For this review, take the finished solid that the model builds, in its own axes (mm). Face numbers are marked on the shaded views. A direction names the side the tool comes from. Round coordinates to 2 decimals unless told otherwise and drop trailing zeros. Order: outer loops, then holes, each group sorted by start corner. A loop starts at its lowest first (then second) coordinate and runs counter-clockwise, first axis right, second up. Notation, with made-up numbers: (47.5, -34) - (90.5, -34) arc R17 ccw to (90.5, -2) - close; hole circle Ø4 at (42, 52). An arc over 180 degrees is marked (long way). One line per question, with ' | ' between items.
```python
from build123d import *

# Parameters (mm, degrees)
SKETCH_1_R                   = 15
EXTRUDE_1_DEPTH              = 5
SKETCH_1_5_R                 = 12
SKETCH_1_5_R_2               = 9.125
EXTRUDE_2_DEPTH              = 20
HOLE_WIZARD_M3_1_D           = 3.4
HOLE_WIZARD_M3_1_CSINK_D     = 6.6
HOLE_WIZARD_M3_1_CSINK_ANGLE = 90
SKETCH1_R                    = 3.25
CUT_EXTRUDE1_DEPTH           = 16
CUT_EXTRUDE1_DEPTH_BACK      = 16
M3_CLEARANCE_HOLE1_D         = 3.4
M3_CLEARANCE_HOLE1_DEPTH     = 35
M3_CLEARANCE_HOLE1_TIP       = 1.021463052


with BuildPart() as part:
    # 草图1 → 凸台-拉伸1 (new body)
    with BuildSketch(Plane(origin=(0, 0, 0), x_dir=(0, 0, -1), z_dir=(1, 0, 0))):
        Circle(SKETCH_1_R)
    extrude(amount=EXTRUDE_1_DEPTH)

    # 草图1<5> → 凸台-拉伸2 (add)
    with BuildSketch(Plane(origin=(0, 0, 0), x_dir=(0, 0, -1), z_dir=(1, 0, 0))):
        Circle(SKETCH_1_5_R)
        Circle(SKETCH_1_5_R_2, mode=Mode.SUBTRACT)
    extrude(amount=EXTRUDE_2_DEPTH)

    # M3 十字槽沉头木螺钉的锥形沉头孔1 (through all)
    with Locations(Plane(origin=(5, 0, 0), x_dir=(0, 0, 1), z_dir=(1, 0, 0))):
        with Locations((0, -5), (-5, 0), (0, 5), (5, 0)):
            CounterSinkHole(HOLE_WIZARD_M3_1_D / 2, HOLE_WIZARD_M3_1_CSINK_D / 2, counter_sink_angle=HOLE_WIZARD_M3_1_CSINK_ANGLE)

    # Sketch1 → Cut-Extrude1 (cut, two sides)
    with BuildSketch(Plane.XY) as cut_extrude1_sk:
        with Locations((12.5, 0)):
            Circle(SKETCH1_R)
    extrude(amount=CUT_EXTRUDE1_DEPTH, mode=Mode.SUBTRACT)
    extrude(cut_extrude1_sk.sketch, amount=-CUT_EXTRUDE1_DEPTH_BACK, mode=Mode.SUBTRACT)

    # M3 Clearance Hole1
    with Locations(Plane(origin=(0, -12, 0), x_dir=(-1, 0, 0), z_dir=(0, -1, 0))):
        with Locations((-12, 0)):
            Hole(M3_CLEARANCE_HOLE1_D / 2, depth=M3_CLEARANCE_HOLE1_DEPTH)
            with Locations((0, 0, -(M3_CLEARANCE_HOLE1_DEPTH + M3_CLEARANCE_HOLE1_TIP / 2))):  # 118° drill point
                Cone(0, M3_CLEARANCE_HOLE1_D / 2, M3_CLEARANCE_HOLE1_TIP, mode=Mode.SUBTRACT)


solid = part.part
```
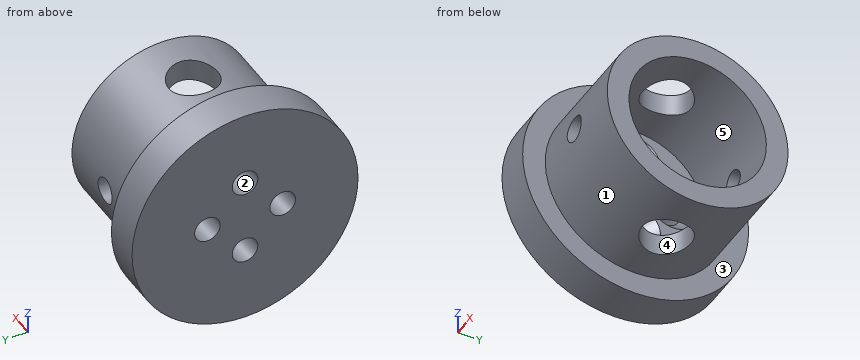
(1) For the marked faces 4 and 5, list the 3-axis set-ups (+Z, -Z, +X, -X, +Y, -Y) from which the entire face can be reached by the end or side of a thin tool; tool diameter is ignored.
Output values:
face 4: +Z, -Z | face 5: +X
(2) Insertion check: pin 1 (12 mm diameter, centred on x = 12.5, z = 4.5, fed in from -Y); pin 2 (16.5 mm diameter, centred on y = 0, z = 0, fed in from +X); pin 3 (4 mm diameter, centred on x = 12, z = 0, fed in from +Y). Each pin has a flat end and moves straight along its axis. Give the tip position at first contact, or say it passes through.
Output values:
pin 1: y = -12 | pin 2: x = 5 | pin 3: y = 12
(3) We need section C-C on x = 13. State the section outline as (y, z) points (3 decimals).
Output values:
outline: (-11.921, -1.375) arc R12 ccw to (-3.211, -11.562) - (-3.211, -8.541) arc R9.125 cw to (-9.021, -1.375) - close; (-11.921, 1.375) - (-9.021, 1.375) arc R9.125 cw to (-3.211, 8.541) - (-3.211, 11.562) arc R12 ccw to start; (3.211, -11.562) arc R12 ccw to (11.921, -1.375) - (9.021, -1.375) arc R9.125 cw to (3.211, -8.541) - close; (3.211, 8.541) arc R9.125 cw to (9.021, 1.375) - (11.921, 1.375) arc R12 ccw to (3.211, 11.562) - close
(4) We need section D-D on x = 3. State the section outline as (y, z) points.
Output values:
outline: circle Ø30 at (0, 0); hole circle Ø3.4 at (-5, 0); hole circle Ø3.4 at (0, -5); hole circle Ø3.4 at (0, 5); hole circle Ø3.4 at (5, 0)
(5) We need section A-A on z = 0. Give the number of separate pieces and of enclosed holes in the cut face, plus the area to 3 significant figures.
Output values:
separate pieces: 5 | enclosed holes: 0 | area: 178 mm^2
(6) For probe 1 along Y at (x, z) = (1.25, 0); probe 2 along X at (y, z) = (0, -10.25); probe 3 along Y at (x, z) = (15.25, 0) (3 decimals), list the stretches that pass through material, from the lowest coordinate up. Write a range as [from, to].
Output values:
probe 1: [-15, -6.7], [-3.3, 3.3], [6.7, 15] | probe 2: [0, 9.25], [15.75, 20] | probe 3: [-12, -9.125], [9.125, 12]
(7) Mouldability with a two-part tool opening along Z and no side actions: class the marked faces 1, 2 and 3 as released by +Z, released by -Z, zero draft, split by the parting line, or undercut.
Output values:
face 1: split by the parting line | face 2: undercut | face 3: zero draft
